Design review of the part built by this model. Coordinates are the model's own, in mm. A direction names the side the tool comes from. Coordinates: 2 decimals unless noted, no trailing zeros. Write each loop counter-clockwise with the first axis right and the second up, starting at its lowest first coordinate (ties: lowest second). Pieces come first, ordered by that corner, then holes. Notation, with made-up numbers: (50.25, 87.25) - (94.25, 87.25) arc R12 cw to (94.25, 98.25) - close; hole circle Ø10 at (86.5, -0.75). An arc over 180 degrees is marked (long way). One line per item, written item: value.
from build123d import *

# Parameters (mm, degrees)
F0_R     = 11
F1_DEPTH = 2
F2_R     = 9.5
F3_DEPTH = 1
F4_R     = 5
F5_DEPTH = 1.7
F6_R     = 3.05
F7_DEPTH = 5
F8_R     = 1.5
F9_DEPTH = 3
F10_R    = 0.5


with BuildPart() as f1:
    # F0 (on Top) → F1 (new body)
    with BuildSketch(Plane.XY):
        Circle(F0_R)
    extrude(amount=F1_DEPTH)

    # F2 (on face) → F3 (cut)
    with BuildSketch(Plane.XY.offset(2)):
        Circle(F2_R)
    extrude(amount=-F3_DEPTH, mode=Mode.SUBTRACT)

    # F4 (on face) → F5 (join)
    with BuildSketch(Plane.XY.offset(1)):
        Circle(F4_R)
    extrude(amount=F5_DEPTH)

    # F6 (on face) → F7 (join)
    with BuildSketch(Plane.XY.offset(2.7)):
        Circle(F6_R)
    extrude(amount=F7_DEPTH)

    # F8 (on face) → F9 (cut)
    with BuildSketch(Plane.XY.offset(7.7)):
        Circle(F8_R)
    extrude(amount=-F9_DEPTH, mode=Mode.SUBTRACT)

    # F10
    f10_edges = [f1.edges().sort_by_distance(p)[0] for p in [
        (-9.5, 0, 2),
        (-11, 0, 2),
        (-3.05, 0, 7.7),
        (-5, 0, 2.7),
    ]]
    fillet(f10_edges, radius=F10_R)


solid = f1.part
1. Consider section A-A, the plane y = 0. Write out the cut boundary in (x, z).
Answer block:
outline: (-11, 0) - (11, 0) - (11, 1.5) arc R0.5 ccw to (10.5, 2) - (10, 2) arc R0.5 ccw to (9.5, 1.5) - (9.5, 1) - (5, 1) - (5, 2.2) arc R0.5 ccw to (4.5, 2.7) - (3.05, 2.7) - (3.05, 7.2) arc R0.5 ccw to (2.55, 7.7) - (1.5, 7.7) - (1.5, 4.7) - (-1.5, 4.7) - (-1.5, 7.7) - (-2.55, 7.7) arc R0.5 ccw to (-3.05, 7.2) - (-3.05, 2.7) - (-4.5, 2.7) arc R0.5 ccw to (-5, 2.2) - (-5, 1) - (-9.5, 1) - (-9.5, 1.5) arc R0.5 ccw to (-10, 2) - (-10.5, 2) arc R0.5 ccw to (-11, 1.5) - close
2. Consider section C-C, the plane z = 3.5. Write out the cut boundary in (x, y), then the cut area to 3 significant figures.
Answer block:
outline: circle Ø6.1 at (0, 0)
area: 29.2 mm^2
3. Mouldability with a two-part tool opening along Y and no side actions: class faces 3 (the face through (-3.047, 0.134, 4.918)), 4 (the face through (0, 0, 0)), 5 (the face through (0, 0, 4.7)) as released by +Y, released by -Y, zero draft, split by the parting line, or undercut.
Answer block:
face 3: split by the parting line
face 4: zero draft
face 5: undercut
4. Insertion check: pin 1 Ø1 at (y, z) = (-2, 1) entering from +X; pin 2 Ø12 at (x, y) = (4.5, 8.5) entering from +Z; pin 3 Ø3 at (x, z) = (7.5, 1.5) entering from -Y; pin 4 Ø2 at (x, y) = (2, -0.5) entering from -Z. Each pin has a flat end and moves straight along its axis. Give the tip position at first contact, or say it passes through.
Answer block:
pin 1: stops at x = 10.9
pin 2: stops at z = 2.7
pin 3: stops at y = -9.22
pin 4: stops at z = 0
5. Wall thickness on line 1 along Y through (x, z) = (0, 1.1); line 2 along Y through (x, z) = (0, 6.65); line 3 along Z through (x, y) = (-2, -10): over which ranges is each line inside the solid? List them lowest first.
Answer block:
line 1: y = -11 to -9.5, -5 to 5, 9.5 to 11
line 2: y = -3.05 to -1.5, 1.5 to 3.05
line 3: z = 0 to 2
6. For faces 1 (the face through (-1.5, 0.07, 6.22)), 2 (the face through (2, 0, 7.7)), list the 3-axis set-ups (+Z, -Z, +X, -X, +Y, -Y) from which the entire face can be reached by the end or side of a thin tool; tool diameter is ignored.
Answer block:
face 1: +Z
face 2: +Z, +X, -X, +Y, -Y
